Build history of the part. All positions in model axes, mm. A direction names the side the tool comes from. Coordinates: 2 decimals unless noted, no trailing zeros. Order: outer loops, then holes, each group sorted by start corner. A loop starts at its lowest first (then second) coordinate and runs counter-clockwise, first axis right, second up. Notation, with made-up numbers: M 11.5,-35.75 L 38.5,-35.75 A25 cw 38.5,1.25 Z; hole C 55,4 d5. An arc over 180 degrees is marked long. Use a Markdown table: item, result. Add a question column.
from build123d import *

# Parameters (mm, degrees)
SKIZZE1_W                            = 50
SKIZZE1_H                            = 3
SKIZZE2_W                            = 10
SKIZZE2_H                            = 2
SCHNITT_LINEAR_AUSTRAGEN1_DEPTH      = 4
SCHNITT_LINEAR_AUSTRAGEN1_DEPTH_BACK = 4


with BuildPart() as part:
    # Skizze1 → Rotation1 (revolve)
    with BuildSketch(Plane.XY):
        with Locations((25, 1.5)):
            Rectangle(SKIZZE1_W, SKIZZE1_H)
    revolve(axis=Axis((0, 0, 0), (1, 0, 0)))

    # Skizze2 → Schnitt-Linear austragen1 (cut, two sides)
    with BuildSketch(Plane.XY) as schnitt_linear_austragen1_sk:
        with Locations((18.5, 3)):
            Rectangle(SKIZZE2_W, SKIZZE2_H)
        with Locations((45, 3)):
            Rectangle(SKIZZE2_W, SKIZZE2_H)
    extrude(amount=SCHNITT_LINEAR_AUSTRAGEN1_DEPTH, mode=Mode.SUBTRACT)
    extrude(schnitt_linear_austragen1_sk.sketch, amount=-SCHNITT_LINEAR_AUSTRAGEN1_DEPTH_BACK, mode=Mode.SUBTRACT)


solid = part.part
(1) Slice it at A-A on z = 0. Give the cut face in (x, y).
(2) Mould opens along X. For faces 4 (the cylindrical face through (25, -3, 0)), 5 (the flat face through (13.5, 2.4, 0)), 6 (the flat face through (40, 2.4, 0)) say: released by +X, released by -X, zero draft, split by the parting line, or undercut.
(3) Slice it at C-C on y = -1.95. Give the cut face in (x, z).
(4) Slice it at B-B on x = 14.5. Give the cut face in (y, z).
(5) Drill centre lines: line 1 along X through (y, z) = (2.5, -0.65); line 2 along Y through (x, z) = (20.5, -0.25); line 3 along Y through (x, z) = (38.5, -0.65). Where is each one in solid material? Low to high. Write a range as from..to.
(6) Slice it at D-D on x = 28. Give the cut face in (y, z), and give its area (3 significant figures).
(7) Which spindle directions (+Z, -Z, +X, -X, +Y, -Y) get a long thin tool onto all of the face, cutting with end or side? Do faces 1 (the flat face through (23.5, 2.4, 0)), 2 (the flat face through (45, 2, 0)), 3 (the flat face through (0, 0, 0)). Say none if no direction does.
(8) Drop flat-ended pins along their axis: P1, Ø0.8, axis at y = 2.5, z = 0.5, coming from the +X side; P2, Ø1.3, axis at x = 19.5, z = 1, coming from the +Y side; P3, Ø1.1, axis at y = 2.5, z = 0, coming from the +X side; P4, Ø1, axis at x = 18, y = -1.5, coming from the +Z side. Give the stop position or say it passes through.
Solutions:
| question | item | result |
|---|---|---|
| 1 | outline | M 0,-3 L 50,-3 L 50,2 L 40,2 L 40,3 L 23.5,3 L 23.5,2 L 13.5,2 L 13.5,3 L 0,3 Z |
| 2 | face 4 | zero draft |
| 2 | face 5 | undercut |
| 2 | face 6 | released by +X |
| 3 | outline | M 0,-2.28 L 50,-2.28 L 50,2.28 L 0,2.28 Z |
| 4 | outline | M 2,-2.24 L 2,2.24 A3 ccw long Z |
| 5 | line 1 | 0..13.5, 23.5..40 |
| 5 | line 2 | -2.99..2 |
| 5 | line 3 | -2.93..2.93 |
| 6 | outline | C 0,0 d6 |
| 6 | area | 28.3 mm² |
| 7 | face 1 | +Z, -Z, +Y |
| 7 | face 2 | +Z, -Z, +X, +Y |
| 7 | face 3 | +Z, -Z, -X, +Y, -Y |
| 8 | P1 | x = 40 |
| 8 | P2 | y = 2 |
| 8 | P3 | x = 50 |
| 8 | P4 | z = 2.83 |
